Build history of the part. All positions in model axes, mm. A direction names the side the tool comes from. Round coordinates to 2 decimals unless told otherwise and drop trailing zeros. Loops run counter-clockwise (first coordinate to the right, second up) from the corner with the lowest first, then second, coordinate; pieces in that order, holes last. Notation, with made-up numbers: (85.5, 56.25) - (143.5, 56.25) arc R26 cw to (143.5, 91.25) - close; hole circle Ø4 at (33.25, 84.5). An arc over 180 degrees is marked (long way). Use a Markdown table: item, result.
from build123d import *

# Parameters (mm, degrees)
BOSS_EXTRUDE1_DEPTH = 3.75
SKETCH2_W           = 4
SKETCH2_H           = 4.100690398
CUT_EXTRUDE1_DEPTH  = 4.5
SKETCH3_W           = 5
SKETCH3_H           = 9.939403745
CUT_EXTRUDE2_DEPTH  = 1.5
CUT_EXTRUDE3_DEPTH  = 1.5


with BuildPart() as part:
    # Sketch1 → Boss-Extrude1 (new body, symmetric)
    with BuildSketch(Plane.XY):
        with BuildLine():
            Line((0, 6), (0, 0))
            Line((0, 0), (3, 0))
            Line((3, 0), (3, 1))
            Line((3, 1), (6, 1))
            Line((6, 1), (6, 0))
            Line((6, 0), (9, 0))
            Line((9, 0), (9, 10))
            Line((9, 10), (7, 10))
            Line((7, 10), (7, 8))
            ThreePointArc((7, 8), (5, 6), (3, 8))
            Line((3, 8), (3, 9))
            Line((3, 9), (1, 9))
            Line((1, 9), (1, 6))
            Line((1, 6), (0, 6))
        make_face()
    extrude(amount=BOSS_EXTRUDE1_DEPTH, both=True)

    # Sketch2 → Cut-Extrude1 (cut)
    with BuildSketch(Plane.XY.offset(3.75)):
        with Locations((3, 8.050345199)):
            Rectangle(SKETCH2_W, SKETCH2_H)
    extrude(amount=-CUT_EXTRUDE1_DEPTH, mode=Mode.SUBTRACT)

    # Sketch3 → Cut-Extrude2 (cut)
    with BuildSketch(Plane.XY.offset(3.75)):
        with Locations((2.5, 4.969701872)):
            Rectangle(SKETCH3_W, SKETCH3_H)
    extrude(amount=-CUT_EXTRUDE2_DEPTH, mode=Mode.SUBTRACT)

    # Sketch4 → Cut-Extrude3 (cut)
    with BuildSketch(Plane.XY.offset(2.25)):
        with BuildLine():
            Line((4, 6), (0, 6))
            Line((0, 6), (0, 2))
            ThreePointArc((0, 2), (2.828427125, 3.171572875), (4, 6))
        make_face()
    extrude(amount=-CUT_EXTRUDE3_DEPTH, mode=Mode.SUBTRACT)


solid = part.part
Q1. Probe line 1 (Y direction, x = 1.25, z = -2.75); line 2 (Z direction, x = 2.5, y = 1); line 3 (Y direction, x = 4, z = 0.25). List the from-to ranges inside material, lowest first.
Results found:
| item | result |
|---|---|
| line 1 | y = 0 to 9 |
| line 2 | z = -3.75 to 2.25 |
| line 3 | y = 1 to 6 |
Q2. Drop flat-ended pins along their axis: pin 1 (0.9 mm diameter, centred on y = 7.5, z = -1.5, fed in from -X); pin 2 (1.6 mm diameter, centred on y = 3, z = 3.5, fed in from -X); pin 3 (2.5 mm diameter, centred on x = 3, y = 8, fed in from +Z); pin 4 (1.5 mm diameter, centred on x = 4.5, y = 7, fed in from +Z). Give the stop position or say it passes through.
Results found:
| item | result |
|---|---|
| pin 1 | stops at x = 1 |
| pin 2 | stops at x = 5 |
| pin 3 | stops at z = -0.75 |
| pin 4 | passes through |
Q3. Cut at D-D, the plane y = 3.25. List the corners of the cut face in (x, z).
Results found:
| item | result |
|---|---|
| outline | (0, -3.75) - (9, -3.75) - (9, 3.75) - (5, 3.75) - (5, 2.25) - (2.9, 2.25) - (2.9, 0.75) - (0, 0.75) - close |
Q4. Cut at C-C, the plane x = 1.25. List the corners of the cut face in (y, z).
Results found:
| item | result |
|---|---|
| outline | (0, -3.75) - (9, -3.75) - (9, -0.75) - (6, -0.75) - (6, 0.75) - (2.2, 0.75) - (2.2, 2.25) - (0, 2.25) - close |
Q5. Cut at B-B, the plane z = 1.5. List the corners of the cut face in (x, y), plus the area to 3 significant figures.
Results found:
| item | result |
|---|---|
| outline | (0, 0) - (3, 0) - (3, 1) - (6, 1) - (6, 0) - (9, 0) - (9, 10) - (7, 10) - (7, 8) arc R2 cw to (5, 6) - (4, 6) arc R4 cw to (0, 2) - close |
| area | 47.3 mm2 |
Q6. Pull direction X, two halves, no side cores. Call faces 1 (the face through (6, 0.5, 0.1)), 2 (the face through (8, 10, 0)), 3 (the face through (2.797, 3.141, 1.51)), 4 (the face through (7, 9, 0)): pulls with the +X half, pulls with the -X half, needs draft (parallel to the pull), parting line crosses it, or undercut.
Results found:
| item | result |
|---|---|
| face 1 | undercut |
| face 2 | needs draft |
| face 3 | pulls with the -X half |
| face 4 | undercut |
Q7. Cut at A-A, the plane y = 8.75. List the corners of the cut face in (x, z), plus the area to 3 significant figures.
Results found:
| item | result |
|---|---|
| outline | (1, -3.75) - (3, -3.75) - (3, -0.75) - (1, -0.75) - close; (7, -3.75) - (9, -3.75) - (9, 3.75) - (7, 3.75) - close |
| area | 21.0 mm2 |
Q8. Which spindle directions (+Z, -Z, +X, -X, +Y, -Y) get a long thin tool onto all of the face, cutting with end or side? Do faces 5 (the face through (3, 2, 2.25)), 6 (the face through (3, 8.5, -2.2)), 7 (the face through (2, 4, 0.75)). Say none if no direction does.
Results found:
| item | result |
|---|---|
| face 5 | +Z, -X, +Y, -Y |
| face 6 | +Z, -Z, +Y |
| face 7 | +Z, -X, +Y |
